```python
from build123d import *

# Parameters (mm, degrees)
F1_DEPTH = 5
F2_R     = 4
F3_DEPTH = 5.001
F4_SIZE  = 0.5


with BuildPart() as f1:
    # F0 (on Right) → F1 (new body)
    with BuildSketch(Plane.YZ):
        Polygon((0, -6.928203), (6, -3.464102), (6, 3.464102), (0, 6.928203), (-6, 3.464102), (-6, -3.464102), align=None)
    extrude(amount=-F1_DEPTH)

    # F2 (on face) → F3 (cut, through all)
    with BuildSketch(Plane.YZ):
        Circle(F2_R)
    extrude(amount=-F3_DEPTH, mode=Mode.SUBTRACT)

    # F4
    f4_edges = [f1.edges().sort_by_distance(p)[0] for p in [
        (0, -4, 0),
        (-2.5, 4, 0),
        (-5, -4, 0),
    ]]
    chamfer(f4_edges, length=F4_SIZE)


solid = f1.part
```
Source: CAD feature listing. Evaluate the final solid. Frame: model axes, mm. Coordinates: 2 decimals unless noted, no trailing zeros. Write each loop counter-clockwise with the first axis right and the second up, starting at its lowest first coordinate (ties: lowest second). Pieces come first, ordered by that corner, then holes. Notation, with made-up numbers: (28, 5) -> (53, 5) arc R7 cw to (53, 16) -> close; hole circle Ø9 at (11, 69.5). An arc over 180 degrees is marked (long way). Return JSON: item names as keys, results as strings. Group by question number.
1) Section query C-C, the plane y = -5. Return loops of the section in (x, z), plus the area to 3 significant figures.
2) Section query D-D, the plane z = 5.5. Return loops of the section in (x, y).
3) Mould query, pull axis Z, two halves, no side actions, for faces 1 (the face through (-2.46, 2.96, -5.22)), 2 (the face through (-2.46, -2.96, 5.22)), 3 (the face through (0, 0, -5)), 4 (the face through (-2.472, -0.867, -3.905)). Classes: +Z half, -Z half, draft (parallel to the pull), parting line (faces both ways), or undercut.
4) Ray query, line 1 along Y through (x, z) = (-2.5, -2); line 2 along Z through (x, y) = (-1.35, 0.25); line 3 along Y through (x, z) = (-1.75, 3). Return the intervals inside material, ascending.
5) Section query A-A, the plane z = 0. Return loops of the section in (x, y).
6) Section query B-B, the plane x = -2.85. Return loops of the section in (y, z), plus the area to 3 significant figures.
From the geometry:
{
 "1": {"outline": "(-5, -4.04) -> (0, -4.04) -> (0, 4.04) -> (-5, 4.04) -> close", "area": "40.4 mm²"},
 "2": {"outline": "(-5, -2.47) -> (0, -2.47) -> (0, 2.47) -> (-5, 2.47) -> close"},
 "3": {"face 1": "-Z half", "face 2": "+Z half", "face 3": "draft", "face 4": "undercut"},
 "4": {"line 1": "-6 to -3.46, 3.46 to 6", "line 2": "-6.78 to -3.99, 3.99 to 6.78", "line 3": "-6 to -2.65, 2.65 to 6"},
 "5": {"outline": "(-5, -6) -> (0, -6) -> (0, -4.5) -> (-0.5, -4) -> (-4.5, -4) -> (-5, -4.5) -> close; (-5, 4.5) -> (-4.5, 4) -> (-0.5, 4) -> (0, 4.5) -> (0, 6) -> (-5, 6) -> close"},
 "6": {"outline": "(-6, -3.46) -> (0, -6.93) -> (6, -3.46) -> (6, 3.46) -> (0, 6.93) -> (-6, 3.46) -> close; hole circle Ø8 at (0, 0)", "area": "74.4 mm²"}
}
